Geometry check sheet. Reference: drawing and pictorial views, mm from the part's lowest x, y, z. Coordinates: 2 decimals unless noted, no trailing zeros. Loops run counter-clockwise (first coordinate to the right, second up) from the corner with the lowest first, then second, coordinate; pieces in that order, holes last.
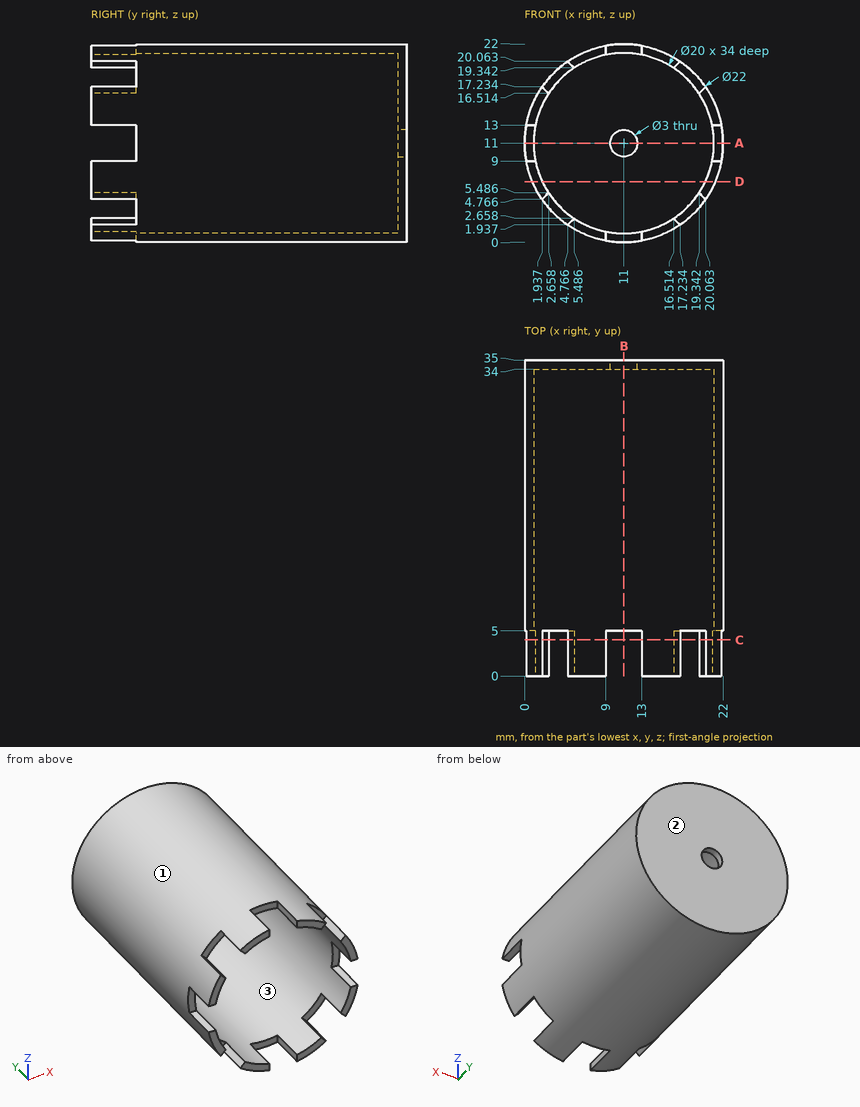
1) Depth check by flat-ended pin: pin 1 (1.1 mm diameter, centred on x = 4, z = 19, fed in from -Y); pin 2 (1.5 mm diameter, centred on x = 3.5, y = 5.5, fed in from -Z) (1 decimal); pin 3 (1 mm diameter, centred on x = 13, y = 14, fed in from +Z). Enter the tip coordinate at first touch or a pass-through.
Data:
pin 1: stops at y = 5
pin 2: stops at z = 2.3
pin 3: stops at z = 21.9
2) Section check C-C on y = 4. Count the separate pieces of the cut face and the enclosed holes in it.
Data:
separate pieces: 8
enclosed holes: 0
3) Section check B-B on x = 11. Record the cut outline in (y, z).
Data:
outline: (5, 0) - (35, 0) - (35, 9.5) - (34, 9.5) - (34, 1) - (5, 1) - close; (5, 21) - (34, 21) - (34, 12.5) - (35, 12.5) - (35, 22) - (5, 22) - close
4) Material ranges on probe 1 along X at (y, z) = (24, 11); probe 2 along X at (y, z) = (34.6, 11), recorded low to high.
Data:
probe 1: x = 0 to 1, 21 to 22
probe 2: x = 0 to 9.5, 12.5 to 22
5) Section check A-A on z = 11. Record the cut outline in (x, y).
Data:
outline: (0, 5) - (1, 5) - (1, 34) - (9.5, 34) - (9.5, 35) - (0, 35) - close; (12.5, 34) - (21, 34) - (21, 5) - (22, 5) - (22, 35) - (12.5, 35) - close
6) Mould release check, pull along X, two halves, no side actions. Record for the marked faces 1, 2 and 3: +X half, -X half, draft (parallel to the pull), parting line (faces both ways), or undercut.
Data:
face 1: parting line
face 2: draft
face 3: undercut
7) Section check D-D on z = 6.75. Record the cut outline in (x, y) (1 decimal).
Data:
outline: (0.9, 0) - (1.9, 0) - (1.9, 34) - (20.1, 34) - (20.1, 0) - (21.1, 0) - (21.1, 35) - (0.9, 35) - close
